```python
from build123d import *

# Parameters (mm, degrees)
SKETCH1_R           = 47.5
BOSS_EXTRUDE1_DEPTH = 2
SKETCH2_R           = 42.5
BOSS_EXTRUDE2_DEPTH = 1.5
BOSS_EXTRUDE2_TAPER = 2
SKETCH5_R           = 10
CUT_EXTRUDE1_DEPTH  = 4
CHAMFER1_SIZE       = 1
SKETCH7_R           = 47.5
SKETCH7_R_2         = 45.6
BOSS_EXTRUDE3_DEPTH = 4
FILLET2_R           = 1


with BuildPart() as part:
    # Sketch1 → Boss-Extrude1 (new body)
    with BuildSketch(Plane(origin=(0, 0, 0), x_dir=(1, 0, 0), z_dir=(0, 1, 0))):
        Circle(SKETCH1_R)
    extrude(amount=BOSS_EXTRUDE1_DEPTH)

    # Sketch2 → Boss-Extrude2 (add)
    with BuildSketch(Plane.XZ):
        Circle(SKETCH2_R)
    extrude(amount=BOSS_EXTRUDE2_DEPTH, taper=BOSS_EXTRUDE2_TAPER)

    # Sketch5 → Cut-Extrude1 (cut)
    with BuildSketch(Plane(origin=(0, 2, 0), x_dir=(1, 0, 0), z_dir=(0, 1, 0))):
        Circle(SKETCH5_R)
    extrude(amount=-CUT_EXTRUDE1_DEPTH, mode=Mode.SUBTRACT)

    # Chamfer1
    chamfer1_edges = [part.edges().sort_by_distance(p)[0] for p in [
        (-10, -1.5, 0),
        (-10, 2, 0),
    ]]
    chamfer(chamfer1_edges, length=CHAMFER1_SIZE)

    # Sketch7 → Boss-Extrude3 (add)
    with BuildSketch(Plane.XZ):
        Circle(SKETCH7_R)
        Circle(SKETCH7_R_2, mode=Mode.SUBTRACT)
    extrude(amount=BOSS_EXTRUDE3_DEPTH)

    # Fillet2
    fillet2_edges = [part.edges().sort_by_distance(p)[0] for p in [
        (-47.5, 2, 0),
    ]]
    fillet(fillet2_edges, radius=FILLET2_R)


solid = part.part
```
Geometry check sheet. Reference: the model listing, model coordinates, mm. A direction names the side the tool comes from. Coordinates: 2 decimals unless noted, no trailing zeros. Order: outer loops, then holes, each group sorted by start corner. A loop starts at its lowest first (then second) coordinate and runs counter-clockwise, first axis right, second up. Notation, with made-up numbers: M 5.5,15.5 L 23.5,15.5 A23 ccw 23.5,37.5 Z; hole C 82.25,35.25 d5. An arc over 180 degrees is marked long. One line per question, with ' | ' between items. Start each with the question number.
Item 1: Cross-section at A-A on x = 0. Enter the section's corners in (y, z).
Item 2: Material ranges on L1, parallel to Z at x = -34.5, y = -0.2; L2, parallel to X at y = -0.8, z = 36.5; L3, parallel to X at y = -0.45, z = -27, recorded low to high. Write a range as [from, to].
Item 3: Draft check along Z on faces 3 (the flat face through (10, 2, 10)), 4 (the flat face through (9, -1.5, -9)), 5 (the cylindrical face through (-10.3, -1.46, -46.37)). Enter one of: pulls with the +Z half, pulls with the -Z half, needs draft (parallel to the pull), parting line crosses it, or undercut.
Item 4: Gauge pin test, flat ends, axial feed: pin 1 (1 mm diameter, centred on x = 0, y = -1, fed in from -Z); pin 2 (1.5 mm diameter, centred on x = -16.5, y = -3, fed in from -Z); pin 3 (1 mm diameter, centred on y = -2, z = 1.5, fed in from +X); pin 4 (23 mm diameter, centred on x = 0, z = 0, fed in from +Y). Record the tip position at first contact, or that the pin passes through.
Item 5: Set-up check for faces 1 (the flat face through (-42.4, -4, 17.8)), 2 (the flat face through (30.2, 0, 30.2)): record each of +Z, -Z, +X, -X, +Y, -Y from which the full face is reachable in a straight line by a thin tool's end or side.
Item 6: Cross-section at B-B on y = -2.65. Enter the section's corners in (x, z).
Findings:
1) outline: M -4,-47.5 L 1,-47.5 A1 ccw 2,-46.5 L 2,-11 L 1,-10 L -0.5,-10 L -1.5,-11 L -1.5,-42.45 L 0,-42.5 L 0,-45.6 L -4,-45.6 Z; M -4,45.6 L 0,45.6 L 0,42.5 L -1.5,42.45 L -1.5,11 L -0.5,10 L 1,10 L 2,11 L 2,46.5 A1 ccw 1,47.5 L -4,47.5 Z
2) L1: z = [-32.65, -29.82], [-24.81, 24.81], [29.82, 32.65] | L2: x = [-30.4, -27.33], [-21.72, 21.72], [27.33, 30.4] | L3: x = [-39.08, -36.75], [-32.8, 32.8], [36.75, 39.08]
3) face 3: needs draft | face 4: undercut | face 5: parting line crosses it
4) pin 1: stops at z = -47.5 | pin 2: stops at z = -44.81 | pin 3: stops at x = 47.49 | pin 4: stops at y = 2
5) face 1: +Z, -Z, +X, -X, -Y | face 2: -Y
6) outline: C 0,0 d95; hole C 0,0 d91.2
